For this review, take the finished solid that the model builds, in its own axes (mm). Face numbers are marked on the shaded views. A direction names the side the tool comes from. Coordinates: 2 decimals unless noted, no trailing zeros. Loops run counter-clockwise (first coordinate to the right, second up) from the corner with the lowest first, then second, coordinate; pieces in that order, holes last. Notation, with made-up numbers: (82.5, -37) -> (111.5, -37) arc R15 ccw to (111.5, -15) -> close; hole circle Ø11 at (-30, -31.75). An arc over 180 degrees is marked (long way). One line per item, written item: value.
from build123d import *

# Parameters (mm, degrees)
SKETCH_1_W          = 40.5
SKETCH_1_H          = 41.1
EXTRUDE_1_DEPTH     = 20
SKETCH_2_W          = 20
SKETCH_2_H          = 2.75
EXTRUDE_2_DEPTH     = 6.2
SKETCH_3_R          = 2
CUT_EXTRUDE_1_DEPTH = 6.2
SKETCH_4_R          = 3
EXTRUDE_3_DEPTH     = 4


with BuildPart() as part:
    # 草图1 → 凸台-拉伸1 (new body)
    with BuildSketch(Plane.XY):
        Rectangle(SKETCH_1_W, SKETCH_1_H)
    extrude(amount=-EXTRUDE_1_DEPTH)

    # 草图2 → 凸台-拉伸2 (add)
    with BuildSketch(Plane(origin=(20.25, 0, 0), x_dir=(0, 0, -1), z_dir=(1, 0, 0))):
        with Locations((10, 8.825)):
            Rectangle(SKETCH_2_W, SKETCH_2_H)
    extrude_2 = extrude(amount=EXTRUDE_2_DEPTH)

    # 草图3 → 切除-拉伸1 (cut)
    with BuildSketch(Plane(origin=(0, 10.2, 0), x_dir=(1, 0, 0), z_dir=(0, 1, 0))):
        with Locations(Location((23.45, 5, 0), (0, 0, 270))):
            Circle(SKETCH_3_R)
        with Locations(Location((23.45, 15, 0), (0, 0, 270))):
            Circle(SKETCH_3_R)
    cut_extrude_1 = extrude(amount=-CUT_EXTRUDE_1_DEPTH, mode=Mode.SUBTRACT)

    # 镜向2: 凸台-拉伸2, 切除-拉伸1 across plane
    add(extrude_2.mirror(Plane(origin=(0, 0, 0), x_dir=(0, 0, 1), z_dir=(1, 0, 0))))
    add(cut_extrude_1.mirror(Plane(origin=(0, 0, 0), x_dir=(0, 0, 1), z_dir=(1, 0, 0))), mode=Mode.SUBTRACT)

    # 草图4 → 凸台-拉伸3 (add)
    with BuildSketch(Plane(origin=(0, 20.55, 0), x_dir=(1, 0, 0), z_dir=(0, 1, 0))):
        with Locations(Location((-10.25, 10, 0), (0, 0, 270))):
            Circle(SKETCH_4_R)
    extrude(amount=EXTRUDE_3_DEPTH)


solid = part.part
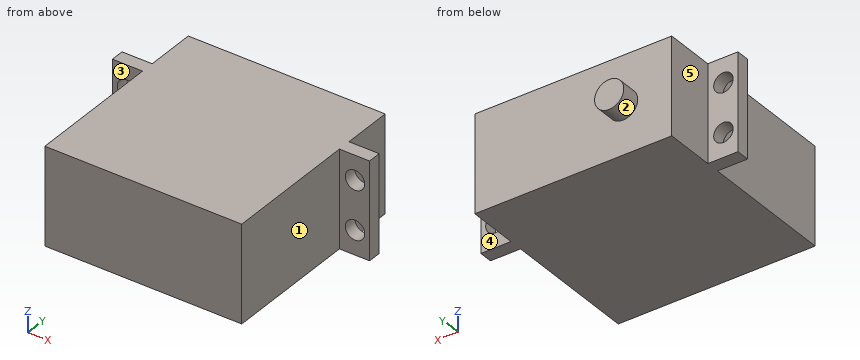
1. Take a section at C-C, the plane z = -10. Give the boundary of the cut face in (x, y).
Return value:
outline: (-26.45, 7.45) -> (-20.25, 7.45) -> (-20.25, -20.55) -> (20.25, -20.55) -> (20.25, 7.45) -> (26.45, 7.45) -> (26.45, 10.2) -> (20.25, 10.2) -> (20.25, 20.55) -> (-7.25, 20.55) -> (-7.25, 24.55) -> (-13.25, 24.55) -> (-13.25, 20.55) -> (-20.25, 20.55) -> (-20.25, 10.2) -> (-26.45, 10.2) -> close
2. For the marked faces 1, 2, 3, 4 and 5, list the 3-axis set-ups (+Z, -Z, +X, -X, +Y, -Y) from which the entire face can be reached by the end or side of a thin tool; tool diameter is ignored.
Return value:
face 1: +Z, -Z, +X, -Y
face 2: +Y
face 3: +Z, -Z, -X, -Y
face 4: +Z, -Z, +X, +Y
face 5: +Z, -Z, -X, +Y
3. Take a section at D-D, the plane y = 1. Give the boundary of the cut face in (x, z), and give its area (3 significant figures).
Return value:
outline: (-20.25, -20) -> (20.25, -20) -> (20.25, 0) -> (-20.25, 0) -> close
area: 810 mm2
4. Take a section at B-B, the plane x = -23.45. Give the boundary of the cut face in (y, z), and give its area (3 significant figures).
Return value:
outline: (7.45, -20) -> (10.2, -20) -> (10.2, -17) -> (7.45, -17) -> close; (7.45, -13) -> (10.2, -13) -> (10.2, -7) -> (7.45, -7) -> close; (7.45, -3) -> (10.2, -3) -> (10.2, 0) -> (7.45, 0) -> close
area: 33.0 mm2
5. Take a section at A-A, the plane z = -15. Give the boundary of the cut face in (x, y), and give its area (3 significant figures).
Return value:
outline: (-26.45, 7.45) -> (-25.45, 7.45) -> (-25.45, 10.2) -> (-26.45, 10.2) -> close; (-21.45, 7.45) -> (-20.25, 7.45) -> (-20.25, -20.55) -> (20.25, -20.55) -> (20.25, 7.45) -> (21.45, 7.45) -> (21.45, 10.2) -> (20.25, 10.2) -> (20.25, 20.55) -> (-20.25, 20.55) -> (-20.25, 10.2) -> (-21.45, 10.2) -> close; (25.45, 7.45) -> (26.45, 7.45) -> (26.45, 10.2) -> (25.45, 10.2) -> close
area: 1,680 mm2
6. Insertion check: pin 1 Ø10 at (x, z) = (-3, -13.5) entering from +Y; pin 2 Ø1.9 at (x, z) = (22, -14) entering from +Y; pin 3 Ø3 at (x, z) = (-23.5, -8) entering from -Y. Each pin has a flat end and moves straight along its axis. Give the tip position at first contact, or say it passes through.
Return value:
pin 1: stops at y = 20.55
pin 2: stops at y = 10.2
pin 3: stops at y = 7.45
7. To check wall thickness, follow probe 1 along X at (y, z) = (8.3, -15); probe 2 along Z at (x, y) = (-23.45, 8.55); probe 3 along Z at (x, y) = (23, 9). State the ranges of each line that lie inside material, in increasing order. Write a range as from..to.
Return value:
probe 1: x = -26.45..-25.45, -21.45..21.45, 25.45..26.45
probe 2: z = -20..-17, -13..-7, -3..0
probe 3: z = -20..-16.95, -13.05..-6.95, -3.05..0
